```python
from build123d import *

# Parameters (mm, degrees)
EXTRUDE_1_DEPTH     = 2
SKETCH_2_R          = 1.65
CUT_EXTRUDE_1_DEPTH = 3.0000001


with BuildPart() as part:
    # 草图1 → 凸台-拉伸1 (new body)
    with BuildSketch(Plane.XY):
        with BuildLine():
            Line((1.423252987, 0), (4.423252987, 0))
            ThreePointArc((4.423252987, 0), (6.082636631, 0.883556575), (6.275860947, 2.753554078))
            ThreePointArc((6.275860947, 2.753554078), (5.811551363, 63.103247136), (46.929512186, 107.280326411))
            ThreePointArc((46.929512186, 107.280326411), (47.763039313, 108.018300592), (48.072882653, 109.087585618))
            Line((48.072882653, 109.087585618), (48.072882653, 111.207813928))
            ThreePointArc((48.072882653, 111.207813928), (47.423208509, 112.683151206), (45.89626257, 113.2))
            Line((45.89626257, 113.2), (30.072910523, 113.2))
            ThreePointArc((30.072910523, 113.2), (28.658696961, 113.785786438), (28.072910523, 115.2))
            Line((28.072910523, 115.2), (28.072910523, 153.5))
            ThreePointArc((28.072910523, 153.5), (28.658696961, 154.914213563), (30.072910523, 155.5))
            Line((30.072910523, 155.5), (46.202994429, 155.5))
            ThreePointArc((46.202994429, 155.5), (47.532372899, 156.128324681), (48.072882653, 157.495763244))
            Line((48.072882653, 157.495763244), (48.072882653, 159.708737404))
            ThreePointArc((48.072882653, 159.708737404), (47.455107078, 161.15423235), (45.983427014, 161.706735824))
            Line((45.983427014, 161.706735824), (27.073474975, 161.706735824))
            ThreePointArc((27.073474975, 161.706735824), (26.186750001, 161.499420632), (25.483856586, 160.920454645))
            ThreePointArc((25.483856586, 160.920454645), (-7.477274918, 84.38693582), (-0.469066984, 1.352601263))
            ThreePointArc((-0.469066984, 1.352601263), (0.260239117, 0.372917108), (1.423252987, 0))
        make_face()
        with BuildLine():
            Line((-3.714345647, 70.477818401), (4.498485812, 107.347765252))
            add(Edge.make_bspline(
                [(4.498485812, 107.347765252), (9.65057542, 132.963079711), (20.376969719, 107.570049249), (18.069358559, 98.588262366)],
                knots=[0, 0, 0, 0, 1, 1, 1, 1], degree=3))
            Line((18.069358559, 98.588262366), (-0.056738646, 68.998256027))
            ThreePointArc((-0.056738646, 68.998256027), (-2.512185077, 68.188921333), (-3.714345647, 70.477818401))
        make_face(mode=Mode.SUBTRACT)
    extrude(amount=EXTRUDE_1_DEPTH)

    # 草图2 → 切除-拉伸1 (cut, through all)
    with BuildSketch(Plane.XY.offset(2)):
        with Locations((43.316196674, 158.665)):
            Circle(SKETCH_2_R)
        with Locations((33.316196674, 158.665)):
            Circle(SKETCH_2_R)
        with Locations((43.316196674, 110.035)):
            Circle(SKETCH_2_R)
        with Locations((33.316196674, 110.035)):
            Circle(SKETCH_2_R)
    extrude(amount=-CUT_EXTRUDE_1_DEPTH, mode=Mode.SUBTRACT)


solid = part.part
```
Can you work these out from the model? Positions are in its coordinate system, mm. A direction names the side the tool comes from. Round coordinates to 2 decimals unless told otherwise and drop trailing zeros. Loops run counter-clockwise (first coordinate to the right, second up) from the corner with the lowest first, then second, coordinate; pieces in that order, holes last. Notation, with made-up numbers: (40.25, 68) -> (97.25, 68) arc R12 cw to (97.25, 88) -> close; hole circle Ø4 at (42.5, 36). An arc over 180 degrees is marked (long way). One line per item, written item: value. Start each with the question number.
1. For pin 1 (4.5 mm diameter, centred on x = 43.32, y = 110.04, fed in from -Z); pin 2 (2 mm diameter, centred on x = 43.32, y = 158.66, fed in from +Z); pin 3 (1 mm diameter, centred on y = 37, z = 1, fed in from +X); pin 4 (0.6 mm diameter, centred on x = 36.5, z = 1.5, fed in from -Y), each with a flat end and sliding along its axis, tell me the tip position at first contact or that it passes through.
2. If we section it at B-B, the plane y = 93.5: Write out the boundary of the cut face in (x, z).
3. If I drill on probe 1 along X at (y, z) = (103, 1.4); probe 2 along X at (y, z) = (107.5, 0.55); probe 3 along Y at (x, z) = (42.5, 0.9), over which ranges is the centre line in solid material (lowest first)?
4. For faces 5 (the flat face through (15, 87, 2)), 6 (the flat face through (0.335, 88.655, 0.986)), which set-ups out of +Z, -Z, +X, -X, +Y, -Y let a thin tool reach every point of the face, with its end or its side?
5. If we mould it in two halves opening along Y, with no side actions, what happens to faces 1 (the flat face through (15, 87, 0)), 2 (the cylindrical face through (-7.284, 85.549, 0.986)), 3 (the cylindrical face through (42.01, 157.66, 1.01)), 4 (the cylindrical face through (5.502, 62.295, 0.986))? For each: pulls with the +Y half, pulls with the -Y half, needs draft (parallel to the pull), parting line crosses it, or undercut.
6. If we section it at A-A, the plane x = 39.5: Write out the boundary of the cut face in (y, z), then the cut area to 3 significant figures.
7. If we section it at D-D, the plane y = 11: Write out the boundary of the cut face in (x, z).
8. If we section it at C-C, the plane z = 1.65: Give the number of separate pieces and of enclosed holes in the cut face, then the cut area to 3 significant figures.
Calculated:
1. pin 1: stops at z = 0
1. pin 2: passes through
1. pin 3: stops at x = 0.36
1. pin 4: stops at y = 101.16
2. outline: (-5.74, 0) -> (1.41, 0) -> (1.41, 2) -> (-5.74, 2) -> close; (14.95, 0) -> (26.53, 0) -> (26.53, 2) -> (14.95, 2) -> close
3. probe 1: x = -3.38 to 3.53, 18.33 to 39.05
3. probe 2: x = -2.05 to 4.53, 17.61 to 47.29
3. probe 3: y = 105.01 to 108.6, 111.47 to 113.2, 155.5 to 157.23, 160.1 to 161.71
4. face 5: +Z, +X, -X, +Y, -Y
4. face 6: +Z, -Z
5. face 1: needs draft
5. face 2: parting line crosses it
5. face 3: undercut
5. face 4: undercut
6. outline: (103.28, 0) -> (113.2, 0) -> (113.2, 2) -> (103.28, 2) -> close; (155.5, 0) -> (161.71, 0) -> (161.71, 2) -> (155.5, 2) -> close
6. area: 32.3 mm²
7. outline: (-3.46, 0) -> (3.42, 0) -> (3.42, 2) -> (-3.46, 2) -> close
8. separate pieces: 1
8. enclosed holes: 5
8. area: 2,480 mm²
